```python
from build123d import *

# Parameters (mm, degrees)
BOSS_EXTRUDE1_DEPTH = 6.35
SKETCH3_R           = 9.875
BOSS_EXTRUDE3_DEPTH = 2.825
SKETCH7_R           = 9.875
BOSS_EXTRUDE5_DEPTH = 2.825


with BuildPart() as part:
    # Sketch1 → Boss-Extrude1 (new body)
    with BuildSketch(Plane.XY):
        with BuildLine():
            Line((0, 9.081), (2.981324224, 8.551667078))
            Line((2.981324224, 8.551667078), (3.126108811, 9.367127025))
            ThreePointArc((3.126108811, 9.367127025), (3.712801822, 9.150449586), (4.284601924, 8.897067571))
            Line((4.284601924, 8.897067571), (3.940098235, 8.181698289))
            Line((3.940098235, 8.181698289), (6.396509598, 6.411237704))
            Line((6.396509598, 6.411237704), (6.880770815, 7.083122051))
            ThreePointArc((6.880770815, 7.083122051), (7.315350136, 6.633345867), (7.720585889, 6.156961793))
            Line((7.720585889, 6.156961793), (7.099811692, 5.661910891))
            Line((7.099811692, 5.661910891), (8.544787799, 3.000984074))
            Line((8.544787799, 3.000984074), (9.272611772, 3.396217886))
            ThreePointArc((9.272611772, 3.396217886), (9.469003638, 2.802426646), (9.627413133, 2.197394223))
            Line((9.627413133, 2.197394223), (8.853320371, 2.020712601))
            Line((8.853320371, 2.020712601), (9.00066598, -1.003651256))
            Line((9.00066598, -1.003651256), (9.827898246, -0.963348883))
            ThreePointArc((9.827898246, -0.963348883), (9.74720484, -1.583547541), (9.627413133, -2.197394223))
            Line((9.627413133, -2.197394223), (8.853320371, -2.020712601))
            Line((8.853320371, -2.020712601), (7.673851879, -4.809501146))
            Line((7.673851879, -4.809501146), (8.436648941, -5.132112591))
            ThreePointArc((8.436648941, -5.132112591), (8.094852581, -5.655880717), (7.720585889, -6.156961793))
            Line((7.720585889, -6.156961793), (7.099811692, -5.661910891))
            Line((7.099811692, -5.661910891), (4.827137299, -7.66277035))
            Line((4.827137299, -7.66277035), (5.374417845, -8.284398459))
            ThreePointArc((5.374417845, -8.284398459), (4.839215493, -8.607997352), (4.284601924, -8.897067571))
            Line((4.284601924, -8.897067571), (3.940098235, -8.181698289))
            Line((3.940098235, -8.181698289), (1.024348976, -8.998333907))
            Line((1.024348976, -8.998333907), (1.247717382, -9.795857611))
            ThreePointArc((1.247717382, -9.795857611), (0.625112426, -9.855194542), (0, -9.875))
            Line((0, -9.875), (0, -9.081))
            Line((0, -9.081), (-2.981324224, -8.551667078))
            Line((-2.981324224, -8.551667078), (-3.126108811, -9.367127025))
            ThreePointArc((-3.126108811, -9.367127025), (-3.712801822, -9.150449586), (-4.284601924, -8.897067571))
            Line((-4.284601924, -8.897067571), (-3.940098235, -8.181698289))
            Line((-3.940098235, -8.181698289), (-6.396509598, -6.411237704))
            Line((-6.396509598, -6.411237704), (-6.880770815, -7.083122051))
            ThreePointArc((-6.880770815, -7.083122051), (-7.315350136, -6.633345867), (-7.720585889, -6.156961793))
            Line((-7.720585889, -6.156961793), (-7.099811692, -5.661910891))
            Line((-7.099811692, -5.661910891), (-8.544787799, -3.000984074))
            Line((-8.544787799, -3.000984074), (-9.272611772, -3.396217886))
            ThreePointArc((-9.272611772, -3.396217886), (-9.469003638, -2.802426646), (-9.627413133, -2.197394223))
            Line((-9.627413133, -2.197394223), (-8.853320371, -2.020712601))
            Line((-8.853320371, -2.020712601), (-9.00066598, 1.003651256))
            Line((-9.00066598, 1.003651256), (-9.827898246, 0.963348883))
            ThreePointArc((-9.827898246, 0.963348883), (-9.74720484, 1.583547541), (-9.627413133, 2.197394223))
            Line((-9.627413133, 2.197394223), (-8.853320371, 2.020712601))
            Line((-8.853320371, 2.020712601), (-7.673851879, 4.809501146))
            Line((-7.673851879, 4.809501146), (-8.436648941, 5.132112591))
            ThreePointArc((-8.436648941, 5.132112591), (-8.094852581, 5.655880717), (-7.720585889, 6.156961793))
            Line((-7.720585889, 6.156961793), (-7.099811692, 5.661910891))
            Line((-7.099811692, 5.661910891), (-4.827137299, 7.66277035))
            Line((-4.827137299, 7.66277035), (-5.374417845, 8.284398459))
            ThreePointArc((-5.374417845, 8.284398459), (-4.839215493, 8.607997352), (-4.284601924, 8.897067571))
            Line((-4.284601924, 8.897067571), (-3.940098235, 8.181698289))
            Line((-3.940098235, 8.181698289), (-1.024348976, 8.998333907))
            Line((-1.024348976, 8.998333907), (-1.247717382, 9.795857611))
            ThreePointArc((-1.247717382, 9.795857611), (-0.625112426, 9.855194542), (0, 9.875))
            Line((0, 9.875), (0, 9.081))
        make_face()
        with BuildLine():
            Line((2.58926817, 8.059275113), (-2.283002739, 8.151326487))
            ThreePointArc((-2.283002739, 8.151326487), (-5.871524586, 6.097657258), (-8.059275113, 2.58926817))
            Line((-8.059275113, 2.58926817), (-8.151326487, -2.283002739))
            ThreePointArc((-8.151326487, -2.283002739), (-6.097657258, -5.871524586), (-2.58926817, -8.059275113))
            Line((-2.58926817, -8.059275113), (2.283002739, -8.151326487))
            ThreePointArc((2.283002739, -8.151326487), (5.871524586, -6.097657258), (8.059275113, -2.58926817))
            Line((8.059275113, -2.58926817), (8.151326487, 2.283002739))
            ThreePointArc((8.151326487, 2.283002739), (6.097657258, 5.871524586), (2.58926817, 8.059275113))
        make_face(mode=Mode.SUBTRACT)
    extrude(amount=BOSS_EXTRUDE1_DEPTH)

    # Sketch3 → Boss-Extrude3 (add)
    with BuildSketch(Plane.XY.offset(6.35)):
        Circle(SKETCH3_R)
        with BuildLine():
            Line((-2.283002739, 8.151326487), (2.58926817, 8.059275113))
            ThreePointArc((2.58926817, 8.059275113), (6.097657258, 5.871524586), (8.151326487, 2.283002739))
            Line((8.151326487, 2.283002739), (8.059275113, -2.58926817))
            ThreePointArc((8.059275113, -2.58926817), (5.871524586, -6.097657258), (2.283002739, -8.151326487))
            Line((2.283002739, -8.151326487), (-2.58926817, -8.059275113))
            ThreePointArc((-2.58926817, -8.059275113), (-6.097657258, -5.871524586), (-8.151326487, -2.283002739))
            Line((-8.151326487, -2.283002739), (-8.059275113, 2.58926817))
            ThreePointArc((-8.059275113, 2.58926817), (-5.871524586, 6.097657258), (-2.283002739, 8.151326487))
        make_face(mode=Mode.SUBTRACT)
    extrude(amount=BOSS_EXTRUDE3_DEPTH)

    # Sketch7 → Boss-Extrude5 (add)
    with BuildSketch(Plane(origin=(0, 0, 0), x_dir=(-1, 0, 0), z_dir=(0, 0, -1))):
        Circle(SKETCH7_R)
        with BuildLine():
            Line((-2.58926817, 8.059275113), (2.283002739, 8.151326487))
            ThreePointArc((2.283002739, 8.151326487), (5.871524586, 6.097657258), (8.059275113, 2.58926817))
            Line((8.059275113, 2.58926817), (8.151326487, -2.283002739))
            ThreePointArc((8.151326487, -2.283002739), (6.097657258, -5.871524586), (2.58926817, -8.059275113))
            Line((2.58926817, -8.059275113), (-2.283002739, -8.151326487))
            ThreePointArc((-2.283002739, -8.151326487), (-5.871524586, -6.097657258), (-8.059275113, -2.58926817))
            Line((-8.059275113, -2.58926817), (-8.151326487, 2.283002739))
            ThreePointArc((-8.151326487, 2.283002739), (-6.097657258, 5.871524586), (-2.58926817, 8.059275113))
        make_face(mode=Mode.SUBTRACT)
    extrude(amount=BOSS_EXTRUDE5_DEPTH)


solid = part.part
```
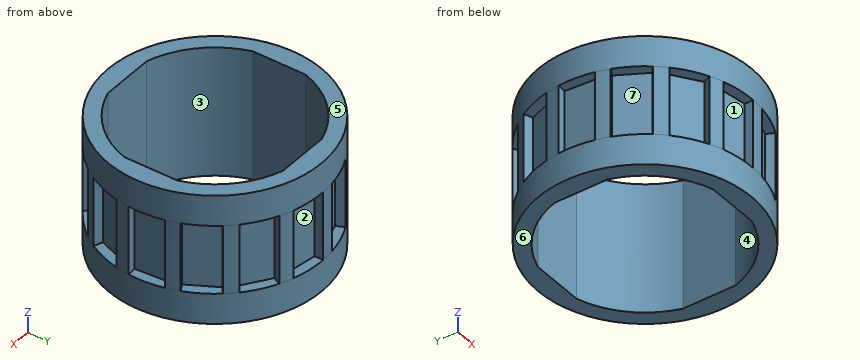
Design review of the part built by this model. Coordinates are the model's own, in mm. Face numbers are marked on the shaded views. A direction names the side the tool comes from. Coordinates: 2 decimals unless noted, no trailing zeros. Write each loop counter-clockwise with the first axis right and the second up, starting at its lowest first coordinate (ties: lowest second). Pieces come first, ordered by that corner, then holes. Notation, with made-up numbers: M 70,44 L 81,44 A29 cw 81,70 Z; hole C -19,59.25 d7. An arc over 180 degrees is marked long. Answer as a JSON object with one key per item and string values.
Item 1: Draft analysis for pull direction Z (two halves, no side actions). For the marked faces 4, 5, 6 and 7, state which applies: pulls with the +Z half, pulls with the -Z half, needs draft (parallel to the pull), parting line crosses it, or undercut.
Outcome:
{"face 4": "needs draft", "face 5": "pulls with the +Z half", "face 6": "pulls with the -Z half", "face 7": "undercut"}
Item 2: Machinability: for the marked faces 1, 2 and 3, which of the approach directions +Z, -Z, +X, -X, +Y, -Y give a long, thin tool a straight path to every point of the face, cutting with its end or side? Answer none if there is none.
Outcome:
{"face 1": "-Y", "face 2": "+Y", "face 3": "+Z, -Z"}
Item 3: Add section C-C, the plane y = -4. Give the boundary of the cut face in (x, z) (3 decimals), and give its area (3 significant figures).
Outcome:
{"outline": "M -9.029,-2.825 L -7.46,-2.825 L -7.46,9.175 L -9.029,9.175 L -9.029,6.35 L -8.002,6.35 L -8.002,0 L -9.029,0 Z; M 7.46,-2.825 L 9.029,-2.825 L 9.029,0 L 8.016,0 L 8.016,6.35 L 9.029,6.35 L 9.029,9.175 L 7.46,9.175 Z", "area": "24.7 mm²"}
Item 4: Add section A-A, the plane z = 8.75. Give the boundary of the cut face in (x, y) (3 decimals), and give its area (3 significant figures).
Outcome:
{"outline": "C 0,0 d19.75; hole M -8.151,-2.283 A8.465 ccw -2.589,-8.059 L 2.283,-8.151 A8.465 ccw 8.059,-2.589 L 8.151,2.283 A8.465 ccw 2.589,8.059 L -2.283,8.151 A8.465 ccw -8.059,2.589 Z", "area": "85.9 mm²"}
Item 5: Add section B-B, the plane x = -5.75. Give the boundary of the cut face in (y, z) (3 decimals).
Outcome:
{"outline": "M -8.028,-2.825 L -6.212,-2.825 L -6.212,9.175 L -8.028,9.175 L -8.028,6.35 L -6.877,6.35 L -6.877,0 L -8.028,0 Z; M 6.212,-2.825 L 8.028,-2.825 L 8.028,0 L 6.85,0 L 6.85,6.35 L 8.028,6.35 L 8.028,9.175 L 6.212,9.175 Z"}
Item 6: Insertion check: pin 1 Ø3 at (x, z) = (2.5, 2.5) entering from -Y; pin 2 Ø3 at (y, z) = (1, 2.5) entering from +X; pin 3 Ø3 at (x, z) = (3.5, -1) entering from -Y. Each pin has a flat end and moves straight along its axis. Give the tip position at first contact, or say it passes through.
Outcome:
{"pin 1": "y = -9.82", "pin 2": "x = 9.63", "pin 3": "y = -9.67"}
Item 7: Wall thickness on probe 1 along Y at (x, z) = (5, 2); probe 2 along Z at (x, y) = (-6.25, -6.75) (3 decimals); probe 3 along Y at (x, z) = (-2, -1.25): over which ranges is each line inside the solid? List them lowest first.
Outcome:
{"probe 1": "-8.52 to -7.86, -7.51 to -6.83, 6.83 to 7.42", "probe 2": "-2.825 to 0, 6.35 to 9.175", "probe 3": "-9.67 to -8.07, 8.15 to 9.67"}
